The model under review builds one solid part; all positions refer to its coordinate system, in mm. A direction names the side the tool comes from. Give positions to 0.01 mm unless a question says otherwise; leave off trailing zeros. Loops run counter-clockwise (first coordinate to the right, second up) from the corner with the lowest first, then second, coordinate; pieces in that order, holes last. Notation, with made-up numbers: (72.5, 47.5) - (116.5, 47.5) arc R30 ccw to (116.5, 69.5) - close; hole circle Ø2 at (18, 40). An arc over 180 degrees is marked (long way). Return JSON: item names as keys, results as strings. Group by question number.
Autodesk Inventor part; units mm, degrees
ref_plane "Work Plane1" through (3.81, 0, 8.636) normal (0, 0, 1) x (1, 0, 0)
ref_plane "Work Plane2" through (11.43, 0, 3.81) normal (0, 0, 1) x (1, 0, 0)
ref_plane "YZ Plane" through (0, 0, 0) normal (1, 0, 0) x (0, 1, 0)
sketch "Sketch1" plane through (0, 0, 0) normal (0, 0, 1) x (1, 0, 0)
  line L0 (0, 25.4) -> (60.96, 25.4)
  line L1 (60.96, 25.4) -> (60.96, 0)
  line L2 (60.96, 0) -> (0, 0)
  line L3 (0, 0) -> (0, 25.4)
  dimension "tmanifold_width" = 60.96
  dimension "tmanifold_depth" = 25.4
extrude "Extrusion1" add sketch "Sketch1" along normal blind 19.05
sketch "Sketch2" plane through (0, 0, 19.05) normal (0, 0, 1) x (1, 0, 0)
  line L0 (60.96, 25.4) -> (60.96, 0)
  line L1 (0, 25.4) -> (60.96, 25.4)
  line L2 (0, 0) -> (0, 25.4)
  line L3 (0, 12.7) -> (60.96, 12.7) construction
  line L4 (3.81, 17.78) -> (3.81, 12.7) construction
  line L5 (11.43, 7.62) -> (11.43, 12.7) construction
  point P0 (19.05, 17.78)
  point P1 (26.67, 7.62)
  point P2 (34.29, 17.78)
  point P3 (41.91, 7.62)
  point P4 (49.53, 17.78)
  point P5 (57.15, 7.62)
  dimension "d5" = 7.62
  dimension "d6" = 7.62
  dimension "d9" = 15.24
  dimension "d14" = 3.81
hole "top 10-32 ports" at (3.81, 17.78, 19.05) at (11.43, 7.62, 19.05) at (26.67, 7.62, 19.05) at (19.05, 17.78, 19.05) at (41.91, 7.62, 19.05) at (34.29, 17.78, 19.05) at (57.15, 7.62, 19.05) at (49.53, 17.78, 19.05) direction (0, 0, -1) diameter 3.9624 depth 6.604
sketch "Sketch3" plane through (0, 0, 0) normal (0, -1, 0) x (1, 0, 0)
  line L0 (60.96, 19.05) -> (0, 19.05)
  line L1 (60.96, 0) -> (0, 0)
  line L2 (1.8288, 12.446) -> (1.8288, 19.05)
  line L3 (5.7912, 12.446) -> (5.7912, 19.05)
  line L4 (5.7912, 12.446) -> (1.8288, 12.446)
  line L5 (9.4488, 12.446) -> (9.4488, 19.05)
  line L6 (13.4112, 12.446) -> (13.4112, 19.05)
  line L7 (13.4112, 12.446) -> (9.4488, 12.446)
  line L8 (3.81, 12.446) -> (3.81, 0) construction
  line L9 (11.43, 12.446) -> (11.43, 0) construction
  circle A0 centre (3.81, 8.636) radius 3.81 construction
  circle A1 centre (11.43, 3.81) radius 3.81 construction
  point P0 (19.05, 8.636)
  point P1 (26.67, 3.81)
  point P2 (34.29, 8.636)
  point P3 (41.91, 3.81)
  point P4 (49.53, 8.636)
  point P5 (57.15, 3.81)
  dimension "d22" = 7.62
  dimension "d25" = 15.24
  dimension "d78" = 8.636
  dimension "d79" = 3.81
hole "front 10-32 ports" at (3.81, 0, 8.636) at (11.43, 0, 3.81) at (19.05, 0, 8.636) at (26.67, 0, 3.81) at (34.29, 0, 8.636) at (41.91, 0, 3.81) at (49.53, 0, 8.636) at (57.15, 0, 3.81) direction (0, 1, 0) diameter 3.9624 depth 6.604
sketch "Sketch4" plane through (0, 25.4, 0) normal (0, 1, 0) x (1, 0, 0)
  circle A0 centre (3.81, -8.636) radius 2.5527
  circle A1 centre (11.43, -3.81) radius 2.5527
  circle A2 centre (19.05, -8.636) radius 2.5527
  circle A3 centre (26.67, -3.81) radius 2.5527
  circle A4 centre (34.29, -8.636) radius 2.5527
  circle A5 centre (41.91, -3.81) radius 2.5527
  circle A6 centre (49.53, -8.636) radius 2.5527
  circle A7 centre (57.15, -3.81) radius 2.5527
  dimension "d76" = 4.826
  dimension "d77" = 9.0197
hole "rear 10-32 ports" at (57.15, 25.4, 3.81) at (49.53, 25.4, 8.636) at (41.91, 25.4, 3.81) at (34.29, 25.4, 8.636) at (26.67, 25.4, 3.81) at (19.05, 25.4, 8.636) at (11.43, 25.4, 3.81) at (3.81, 25.4, 8.636) direction (0, -1, 0) diameter 3.9624 depth 6.604
sketch "Sketch5" plane through (0, 0, 0) normal (0, -1, 0) x (1, 0, 0)
  circle A0 centre (57.15, 3.81) radius 2.5527
  circle A1 centre (49.53, 8.636) radius 2.5527
  circle A2 centre (41.91, 3.81) radius 2.5527
  circle A3 centre (34.29, 8.636) radius 2.5527
  circle A4 centre (26.67, 3.81) radius 2.5527
  circle A5 centre (19.05, 8.636) radius 2.5527
  circle A6 centre (11.43, 3.81) radius 2.5527
  circle A7 centre (3.81, 8.636) radius 2.5527
hole "air channel thru" at (3.81, 0, 8.636) at (11.43, 0, 3.81) at (19.05, 0, 8.636) at (26.67, 0, 3.81) at (34.29, 0, 8.636) at (41.91, 0, 3.81) at (49.53, 0, 8.636) at (57.15, 0, 3.81) direction (0, 1, 0) diameter 1.016 end through all
sketch "Sketch6" plane through (0, 0, 19.05) normal (0, 0, 1) x (1, 0, 0)
  circle A0 centre (49.53, 17.78) radius 2.5527
  circle A1 centre (57.15, 7.62) radius 2.5527
  circle A2 centre (34.29, 17.78) radius 2.5527
  circle A3 centre (41.91, 7.62) radius 2.5527
  circle A4 centre (19.05, 17.78) radius 2.5527
  circle A5 centre (26.67, 7.62) radius 2.5527
  circle A6 centre (11.43, 7.62) radius 2.5527
  circle A7 centre (3.81, 17.78) radius 2.5527
ref_plane "Work Plane1" through (3.81, 0, 8.636) normal (0, 0, 1) x (1, 0, 0)
ref_plane "Work Plane2" through (11.43, 0, 3.81) normal (0, 0, 1) x (1, 0, 0)
hole "Hole5" at (3.81, 17.78, 19.05) at (19.05, 17.78, 19.05) at (34.29, 17.78, 19.05) at (49.53, 17.78, 19.05) direction (0, 0, -1) diameter 1.016 depth 10.414
hole "Hole6" at (11.43, 7.62, 19.05) at (26.67, 7.62, 19.05) at (41.91, 7.62, 19.05) at (57.15, 7.62, 19.05) direction (0, 0, -1) diameter 1.016 depth 15.24
sketch "Sketch7" plane through (0, 0, 0) normal (0, 0, -1) x (-1, 0, 0)
  line L0 (-1.8288, 6.604) -> (-1.8288, 0)
  line L1 (-5.7912, 6.604) -> (-5.7912, 0)
  line L2 (-3.302, 18.796) -> (-3.302, 6.604)
  line L3 (-4.318, 18.796) -> (-4.318, 6.604)
  line L4 (-1.8288, 18.796) -> (-1.8288, 25.4)
  line L5 (-5.7912, 18.796) -> (-5.7912, 25.4)
  line L6 (-1.8288, 18.796) -> (-5.7912, 18.796)
  line L7 (-5.7912, 6.604) -> (-1.8288, 6.604)
  line L8 (-8.8773, 0) -> (-13.9827, 0)
  line L9 (-13.4112, 0.5715) -> (-9.4488, 0.5715)
  line L10 (-13.4112, 6.604) -> (-13.4112, 0)
  line L11 (-9.4488, 6.604) -> (-9.4488, 0)
  line L12 (-10.922, 18.796) -> (-10.922, 6.604)
  line L13 (-11.938, 18.796) -> (-11.938, 6.604)
  line L14 (-9.4488, 18.796) -> (-13.4112, 18.796)
  line L15 (-18.542, 18.796) -> (-18.542, 6.604)
  line L16 (-19.558, 18.796) -> (-19.558, 6.604)
  line L17 (-21.0312, 6.604) -> (-17.0688, 6.604)
  line L18 (-28.6512, 6.604) -> (-24.6888, 6.604)
  line L19 (-36.2712, 6.604) -> (-32.3088, 6.604)
  line L20 (-31.7373, 0) -> (-36.8427, 0)
  line L21 (-43.8912, 6.604) -> (-39.9288, 6.604)
  line L22 (-51.5112, 6.604) -> (-47.5488, 6.604)
  line L23 (-49.022, 18.796) -> (-49.022, 6.604)
  line L24 (-50.038, 18.796) -> (-50.038, 6.604)
  line L25 (-49.022, 18.796) -> (-49.022, 6.604)
  line L26 (-50.038, 18.796) -> (-50.038, 6.604)
  line L27 (-33.782, 18.796) -> (-33.782, 6.604)
  line L28 (-33.782, 18.796) -> (-33.782, 6.604)
  line L29 (-32.3088, 6.604) -> (-32.3088, 0)
  line L30 (-33.782, 18.796) -> (-33.782, 6.604)
  line L31 (-33.782, 18.796) -> (-33.782, 6.604)
  line L32 (-41.402, 18.796) -> (-41.402, 6.604)
  line L33 (-42.418, 18.796) -> (-42.418, 6.604)
  line L34 (-27.178, 18.796) -> (-27.178, 6.604)
  line L35 (-21.0312, 18.796) -> (-21.0312, 25.4)
  line L36 (-27.178, 18.796) -> (-27.178, 6.604)
  line L37 (-42.418, 18.796) -> (-42.418, 6.604)
  line L38 (-36.2712, 18.796) -> (-36.2712, 25.4)
  line L39 (-34.798, 18.796) -> (-34.798, 6.604)
  line L40 (-39.9288, 18.796) -> (-43.8912, 18.796)
  line L41 (-47.5488, 18.796) -> (-51.5112, 18.796)
  line L42 (-55.1688, 18.796) -> (-59.1312, 18.796)
  line L43 (-56.642, 18.796) -> (-56.642, 6.604)
  line L44 (-57.658, 18.796) -> (-57.658, 6.604)
  line L45 (-59.1312, 6.604) -> (-55.1688, 6.604)
  line L46 (-32.3088, 18.796) -> (-36.2712, 18.796)
  line L47 (-26.162, 18.796) -> (-26.162, 6.604)
  line L48 (-24.6888, 18.796) -> (-28.6512, 18.796)
  line L49 (-60.96, 25.4) -> (-60.96, 0)
  line L50 (0, 25.4) -> (-60.96, 25.4)
  line L51 (0, 0) -> (0, 25.4)
  line L52 (-60.96, 0) -> (0, 0)
  line L53 (-28.6512, 6.604) -> (-28.6512, 0)
  line L54 (-24.6888, 6.604) -> (-24.6888, 0)
  line L55 (-36.2712, 6.604) -> (-36.2712, 0)
  line L56 (-39.9288, 6.604) -> (-39.9288, 0)
  line L57 (-43.8912, 6.604) -> (-43.8912, 0)
  line L58 (-47.5488, 6.604) -> (-47.5488, 0)
  line L59 (-51.5112, 6.604) -> (-51.5112, 0)
  line L60 (-55.1688, 6.604) -> (-55.1688, 0)
  line L61 (-59.1312, 6.604) -> (-59.1312, 0)
  line L62 (-39.9288, 18.796) -> (-39.9288, 25.4)
  line L63 (-43.8912, 18.796) -> (-43.8912, 25.4)
  line L64 (-51.5112, 18.796) -> (-51.5112, 25.4)
  line L65 (-55.1688, 18.796) -> (-55.1688, 25.4)
  line L66 (-59.1312, 18.796) -> (-59.1312, 25.4)
  line L67 (-17.0688, 18.796) -> (-21.0312, 18.796)
  line L68 (-17.0688, 18.796) -> (-17.0688, 25.4)
  line L69 (-17.0688, 6.604) -> (-17.0688, 0)
  line L70 (-21.0312, 6.604) -> (-21.0312, 0)
  line L71 (-13.4112, 18.796) -> (-13.4112, 25.4)
  line L72 (-9.4488, 18.796) -> (-9.4488, 25.4)
  circle A0 centre (-34.29, 17.78) radius 2.5527
  circle A1 centre (-19.05, 17.78) radius 2.5527
  circle A2 centre (-3.81, 17.78) radius 2.5527
  circle A3 centre (-11.43, 7.62) radius 2.5527
  circle A4 centre (-26.67, 7.62) radius 2.5527
  circle A5 centre (-41.91, 7.62) radius 2.5527
  circle A6 centre (-49.53, 17.78) radius 2.5527
  circle A7 centre (-57.15, 7.62) radius 2.5527
  line L73 (-32.3088, 18.796) -> (-32.3088, 25.4)
  line L74 (-28.6512, 18.796) -> (-28.6512, 25.4)
  line L75 (-24.6888, 18.796) -> (-24.6888, 25.4)
  line L76 (-13.4112, 6.604) -> (-9.4488, 6.604)
  line L77 (-47.5488, 18.796) -> (-47.5488, 25.4)
  line L78 (-60.96, 12.7) -> (0, 12.7) construction
  line L79 (-30.48, 25.4) -> (-30.48, 0) construction
  point P0 (-9.4488, 0.5715)
  point P1 (-30.48, 12.7)
  point P2 (-15.24, 12.7)
  point P3 (-45.72, 12.7)
  dimension "d68" = 15.24
sketch "Sketch8" plane through (0, 0, 19.05) normal (0, 0, 1) x (1, 0, 0)
  circle A0 centre (49.53, 17.78) radius 2.5527
  circle A1 centre (57.15, 7.62) radius 2.5527
  circle A2 centre (34.29, 17.78) radius 2.5527
  circle A3 centre (41.91, 7.62) radius 2.5527
  circle A4 centre (19.05, 17.78) radius 2.5527
  circle A5 centre (26.67, 7.62) radius 2.5527
  circle A6 centre (11.43, 7.62) radius 2.5527
  circle A7 centre (3.81, 17.78) radius 2.5527
  line L0 (60.96, 25.4) -> (60.96, 0)
  line L1 (0, 25.4) -> (60.96, 25.4)
  line L2 (0, 0) -> (0, 25.4)
  line L3 (60.96, 0) -> (0, 0)
  line L4 (0, 12.7) -> (60.96, 12.7) construction
  line L5 (0, 12.7) -> (60.96, 12.7)
  line L6 (30.48, 0) -> (30.48, 25.4) construction
  line L7 (11.938, 18.796) -> (11.938, 6.604)
  line L8 (10.922, 18.796) -> (10.922, 6.604)
  line L9 (18.542, 18.796) -> (18.542, 6.604)
  line L10 (19.558, 18.796) -> (19.558, 6.604)
  line L11 (26.162, 18.796) -> (26.162, 6.604)
  line L12 (27.178, 18.796) -> (27.178, 6.604)
  line L13 (33.782, 18.796) -> (33.782, 6.604)
  line L14 (34.798, 18.796) -> (34.798, 6.604)
  line L15 (42.418, 18.796) -> (42.418, 6.604)
  line L16 (41.402, 18.796) -> (41.402, 6.604)
  line L17 (49.022, 18.796) -> (49.022, 6.604)
  line L18 (50.038, 18.796) -> (50.038, 6.604)
  point P0 (30.48, 12.7)
  point P1 (45.72, 12.7)
  point P2 (15.24, 12.7)
  dimension "d66" = 30.48
  dimension "d67" = 15.24
hole "Hole7" at (30.48, 12.7, 0) at (15.24, 12.7, 0) at (45.72, 12.7, 0) direction (0, 0, 1) diameter 3.302 depth 12.7 tip angle 118
properties part number "t-manifold ems"
Item 1: Take a section at B-B (x = 40.5). State the section outline as (y, z) points, then the cut area to 3 significant figures.
Item 2: Take a section at A-A (z = 7.5). State how many separate pieces and enclosed holes the cut face has, then the cut area to 3 significant figures.
Item 3: Tool access review of faces 1 (the face through (5.568, 3.348, 7.722)), 2 (the face through (19, 17, 12.446)), 3 (the face through (28.43, 22.05, 4.72)): name each direction out of +Z, -Z, +X, -X, +Y, -Y from which nothing blocks a thin tool from reaching the whole face with its end or side.
Item 4: Mouldability with a two-part tool opening along Z and no side actions: class faces 4 (the face through (35.5, 19.35, 15.7)), 5 (the face through (58, 7, 12.446)), 6 (the face through (26, 18.796, 4)) as +Z half, -Z half, draft (parallel to the pull), parting line (faces both ways), or undercut.
Item 5: For L1, parallel to X at y = 21.75, z = 3.81; L2, parallel to X at y = 7.62, z = 7.5; L3, parallel to Z at x = 34.29, y = 2.5, list the stretches that pass through material, from the lowest coordinate up. Write a range as from..to.
Item 6: For P1, Ø1.2, axis at x = 42.5, y = 8, coming from the +Z side; P2, Ø12, axis at x = 36.5, y = 4, coming from the -Z side; P3, Ø1.6, axis at x = 26.67, z = 3.81, coming from the +Y side; P4, Ø2, axis at x = 4, z = 9.5, coming from the -Y side, all flat-tipped, find the tip position at first contact; note any pin that passes through.
Check sheet entries:
{
 "1": {"outline": "(0, 0) - (25.4, 0) - (25.4, 2.42) - (18.8, 2.42) - (18.8, 5.2) - (25.4, 5.2) - (25.4, 19.05) - (9.01, 19.05) - (9.01, 12.45) - (6.23, 12.45) - (6.23, 19.05) - (0, 19.05) - (0, 5.2) - (6.6, 5.2) - (6.6, 2.42) - (0, 2.42) - close", "area": "429 mm^2"},
 "2": {"separate pieces": "1", "enclosed holes": "7", "area": "1,350 mm^2"},
 "3": {"face 1": "-Y", "face 2": "+Z", "face 3": "+Y"},
 "4": {"face 4": "draft", "face 5": "+Z half", "face 6": "undercut"},
 "5": {"L1": "x = 0..9.45, 13.41..24.69, 28.65..39.93, 43.89..55.17, 59.13..60.96", "L2": "x = 0..10.92, 11.94..26.16, 27.18..41.4, 42.42..56.64, 57.66..60.96", "L3": "z = 0..6.65, 10.62..19.05"},
 "6": {"P1": "stops at z = 12.45", "P2": "stops at z = 0", "P3": "stops at y = 18.8", "P4": "stops at y = 6.6"}
}
